Geometry: final body of the model. Coordinates: model frame, mm. Give positions to 0.01 mm unless a question says otherwise; leave off trailing zeros. Order: outer loops, then holes, each group sorted by start corner. A loop starts at its lowest first (then second) coordinate and runs counter-clockwise, first axis right, second up. Notation, with made-up numbers: (-15.5, 27) -> (-0.5, 27) arc R22 cw to (-0.5, 46) -> close; hole circle Ø11 at (-11, 64). An arc over 180 degrees is marked (long way). Write item = value, one per line.
```python
from build123d import *

# Parameters (mm, degrees)
F0_W         = 228.6
F0_H         = 876.3
F0_R         = 79.375
F0_R_2       = 90.4875
F0_R_3       = 52.3875
F0_R_4       = 73.025
F0_R_5       = 38.1
F0_R_6       = 66.675
F1_DEPTH     = 19.05
F2_DEPTH     = 3.175
F4_R         = 19.04999
F5_T1_DEPTH  = 838.20002
F5_T3_DEPTH  = 32.6603839472
F5_T6_ANGLE  = 90
F5_T8_ANGLE  = 90
F5_T10_ANGLE = 90
F5_T12_ANGLE = 90


# Not quite as in the source:
# - a fillet or chamfer that OpenCascade refuses, or shapes differently, is made with other operations: its cross-section is extruded or revolved along the edge and cut away or added
# - a fillet or chamfer is up to 0.001 mm smaller than in the source, because OpenCascade refuses the exact size


with BuildPart() as f1:
    # F0 (on Front) → F1 (new body)
    with BuildSketch(Plane.XZ):
        with Locations((0, 476.25)):
            Rectangle(F0_W, F0_H)
        with Locations((0, 153.9875)):
            Circle(F0_R, mode=Mode.SUBTRACT)
        with Locations((0, 482.6)):
            Circle(F0_R_2, mode=Mode.SUBTRACT)
        with Locations((33.3502, 635)):
            Circle(F0_R_3, mode=Mode.SUBTRACT)
        with Locations((0, 787.4)):
            Circle(F0_R_2, mode=Mode.SUBTRACT)
        with Locations((0, 787.4)):
            Circle(F0_R_2)
        with Locations((0, 787.4)):
            Circle(F0_R_4, mode=Mode.SUBTRACT)
        with Locations((33.3502, 635)):
            Circle(F0_R_3)
        with Locations((33.3502, 635)):
            Circle(F0_R_5, mode=Mode.SUBTRACT)
        with Locations((0, 482.6)):
            Circle(F0_R_2)
        with Locations((0, 482.6)):
            Circle(F0_R_4, mode=Mode.SUBTRACT)
        with Locations((0, 153.9875)):
            Circle(F0_R)
        with Locations((0, 153.9875)):
            Circle(F0_R_6, mode=Mode.SUBTRACT)
    extrude(amount=-F1_DEPTH)

    # F0 (on Front) → F2 (cut)
    with BuildSketch(Plane.XZ):
        with Locations((0, 787.4)):
            Circle(F0_R_2)
        with Locations((0, 787.4)):
            Circle(F0_R_4, mode=Mode.SUBTRACT)
        with Locations((33.3502, 635)):
            Circle(F0_R_3)
        with Locations((33.3502, 635)):
            Circle(F0_R_5, mode=Mode.SUBTRACT)
        with Locations((0, 482.6)):
            Circle(F0_R_2)
        with Locations((0, 482.6)):
            Circle(F0_R_4, mode=Mode.SUBTRACT)
        with Locations((0, 153.9875)):
            Circle(F0_R)
        with Locations((0, 153.9875)):
            Circle(F0_R_6, mode=Mode.SUBTRACT)
    extrude(amount=-F2_DEPTH, mode=Mode.SUBTRACT)

    # F4 (radius 19.05 in the source; OpenCascade refuses exactly that, so slightly less here)
    f4_edges = [f1.edges().sort_by_distance(p)[0] for p in [
        (0, 0, 914.4),
        (0, 0, 38.1),
    ]]
    fillet(f4_edges, radius=F4_R)

    # F5: chamfer of 12.7 on 2 edges, made by hand

    # F5_s2 → F5_t1 (cut)
    with BuildSketch(Plane.XY.offset(57.14999)):
        Polygon((-101.6, 0), (-114.3, 12.7), (-114.3, 0), align=None)
        Polygon((114.3, 12.7), (101.6, 0), (114.3, 0), align=None)
    extrude(amount=F5_T1_DEPTH, mode=Mode.SUBTRACT)

    # F5_s4 → F5_t3 (cut)
    with BuildSketch(Plane.XZ.offset(-51.7103739472)):
        Polygon((114.3, 901.7), (101.6, 914.4), (114.3, 914.4), align=None)
        Polygon((114.3, 50.8), (101.6, 38.1), (114.3, 38.1), align=None)
        Polygon((-101.6, 38.1), (-114.3, 50.8), (-114.3, 38.1), align=None)
        Polygon((-101.6, 914.4), (-114.3, 901.7), (-114.3, 914.4), align=None)
    extrude(amount=F5_T3_DEPTH, mode=Mode.SUBTRACT)

    # F5_s5 → F5_t6 (revolve, cut)
    with BuildSketch(Plane.XZ.offset(-19.04999)):
        Polygon((114.3, 50.8), (101.6, 38.1), (114.3, 38.1), align=None)
    revolve(axis=Axis((114.3, 19.04999, 57.14999), (-1, 0, 0)), revolution_arc=F5_T6_ANGLE, mode=Mode.SUBTRACT)

    # F5_s7 → F5_t8 (revolve, cut)
    with BuildSketch(Plane.XZ.offset(-19.04999)):
        Polygon((114.3, 901.7), (101.6, 914.4), (114.3, 914.4), align=None)
    revolve(axis=Axis((114.3, 19.04999, 895.35001), (1, 0, 0)), revolution_arc=F5_T8_ANGLE, mode=Mode.SUBTRACT)

    # F5_s9 → F5_t10 (revolve, cut)
    with BuildSketch(Plane.XZ.offset(-19.04999)):
        Polygon((-101.6, 914.4), (-114.3, 901.7), (-114.3, 914.4), align=None)
    revolve(axis=Axis((-114.3, 19.04999, 895.35001), (1, 0, 0)), revolution_arc=F5_T10_ANGLE, mode=Mode.SUBTRACT)

    # F5_s11 → F5_t12 (revolve, cut)
    with BuildSketch(Plane.XZ.offset(-19.04999)):
        Polygon((-101.6, 38.1), (-114.3, 50.8), (-114.3, 38.1), align=None)
    revolve(axis=Axis((-114.3, 19.04999, 57.14999), (-1, 0, 0)), revolution_arc=F5_T12_ANGLE, mode=Mode.SUBTRACT)


solid = f1.part
```
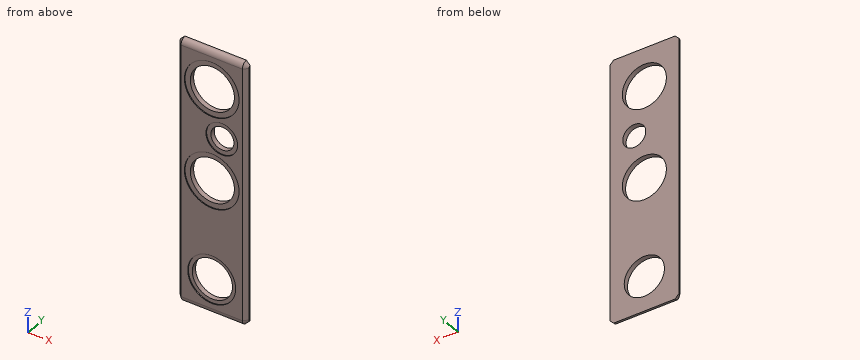
1) Section query A-A (z = 635). Output: boundary loops of the cut face in (x, y) (3 decimals).
Check sheet entries:
outline = (-114.3, 12.7) -> (-101.6, 0) -> (-19.037, 0) -> (-19.037, 3.175) -> (-4.75, 3.175) -> (-4.75, 19.05) -> (-114.3, 19.05) -> close; (71.45, 3.175) -> (85.738, 3.175) -> (85.738, 0) -> (101.6, 0) -> (114.3, 12.7) -> (114.3, 19.05) -> (71.45, 19.05) -> close
2) First-contact query: P1, Ø4, axis at x = -70.5, z = 763, coming from the -Y side (3 decimals); P2, Ø1.5, axis at x = -27, y = 8, coming from the -Z side; P3, Ø2, axis at x = 18, y = 4, coming from the +Z side. Flat tips, straight axial feed; report the tip coordinate or a pass-through.
Check sheet entries:
P1 = 3.175
P2 = 41.12
P3 = 908.21
3) Line query: line 1 (Z direction, x = 0, y = 2.5); line 2 (Z direction, x = -32, y = 16.75); line 3 (Z direction, x = 0, y = 1.7). Output: solid intervals per line, ascending. Write a range as from..to.
Check sheet entries:
line_1 = 47.72..74.61, 233.36..392.11, 573.09..594.6, 675.4..696.91, 877.89..904.78
line_2 = 38.24..95.49, 212.48..416.96, 548.24..721.76, 853.04..914.26
line_3 = 49.28..74.61, 233.36..392.11, 573.09..594.6, 675.4..696.91, 877.89..903.22
4) Section query B-B (x = 54.5). Count the separate pieces of the cut face and the enclosed holes in it, plus the area to 3 significant figures.
Check sheet entries:
separate_pieces = 5
enclosed_holes = 0
area = 9,640 mm²
